Autodesk Inventor part; units mm, degrees
ref_plane "YZ Plane" through (0, 0, 0) normal (1, 0, 0) x (0, 1, 0)
ref_plane "XZ Plane" through (0, 0, 0) normal (0, 1, 0) x (-1, 0, 0)
ref_plane "XY Plane" through (0, 0, 0) normal (0, 0, 1) x (1, 0, 0)
sketch "Sketch4" plane through (0, 0, 0) normal (0, 1, 0) x (-1, 0, 0)
  line L0 (-127, 215.9) -> (127, 215.9)
  line L1 (127, 215.9) -> (127, -215.9)
  line L2 (127, -215.9) -> (-127, -215.9)
  line L3 (-127, -215.9) -> (-127, 215.9)
  line L4 (-127, 215.9) -> (127, -215.9) construction
  line L5 (127, 215.9) -> (-127, -215.9) construction
  point P0 (0, 0)
  dimension "d6" = 431.8
  dimension "d7" = 254
extrude "Plate1" add sketch "Sketch4" against normal blind 6.35
sketch "Sketch5" plane through (120.65, 0, -215.9) normal (1, 0, 0) x (0, -1, 0)
  line L0 (0, 431.8) -> (0, 0)
  line L1 (0, 0) -> (76.2, 0)
  line L2 (76.2, 0) -> (76.2, 431.8)
  line L3 (76.2, 431.8) -> (0, 431.8)
edge flange "Flange1" height 76.2 angle 90 thickness 6.35 bend radius 7.9502 thickness toward (1, 0, 0) relief tear relief width 6.35 relief depth 3.175 corner gap 6.35 corner form 0 edges at (127, 0, 0) (-127, 0, 0) wall of the first edge with corners at (120.65, 0, 215.9) (120.65, 0, -215.9) (120.65, -76.2, -215.9) (120.65, -76.2, 215.9)
bend "Bend1"
corner "Corner1"
sketch "Sketch6" plane through (0, 0, 0) normal (0, 1, 0) x (1, 0, 0)
  circle A0 centre (0, 0) radius 29.083
  dimension "d19" = 58.166
extrude "Cut1" cut sketch "Sketch6" against normal blind 6.35
sketch "Sketch7" plane through (0, 0, 0) normal (0, 1, 0) x (1, 0, 0)
  line L0 (-41.275, -165.1) -> (41.275, -165.1)
  line L1 (41.275, -165.1) -> (41.275, 165.1)
  line L2 (41.275, 165.1) -> (-41.275, 165.1)
  line L3 (-41.275, 165.1) -> (-41.275, -165.1)
  line L4 (-41.275, -165.1) -> (41.275, 165.1) construction
  line L5 (41.275, -165.1) -> (-41.275, 165.1) construction
  line L6 (112.6998, 215.9) -> (-112.6998, 215.9)
  point P0 (0, 0)
  dimension "d22" = 82.55
  dimension "d23" = 50.8
hole "Hole1" at (-41.275, 0, 165.1) at (41.275, 0, 165.1) at (-41.275, 0, -165.1) at (41.275, 0, -165.1) direction (0, -1, 0) diameter 12.7 depth 6.35
fillet "Corner Round1" radius 25.4 4 edges at (-123.825, -76.2, 215.9) (123.825, -76.2, 215.9) (123.825, -76.2, -215.9) (-123.825, -76.2, -215.9)
equation "\"d20\" = Thickness"
equation "\"d29\" = Thickness"
equation "\"d8\" = Thickness"
equation "\"d9\" = BendReliefWidth"
equation "\"d10\" = BendReliefDepth"
equation "\"d11\" = MinimumRemnant"
equation "\"d12\" = TransitionRadius"
equation "\"d15\" = BendRadius"
equation "\"d16\" = CornerReliefSize"
equation "\"d17\" = GapSize"
equation "\"d18\" = JacobiRadiusSize"
equation "\"BendReliefWidth\" = Thickness"
equation "\"BendReliefDepth\" = 0.5 * Thickness"
equation "\"CornerReliefSize\" = 4 * Thickness"
equation "\"MinimumRemnant\" = 2 * Thickness"
equation "\"TransitionRadius\" = BendRadius"
equation "\"JacobiRadiusSize\" = Thickness"
equation "\"GapSize\" = Thickness"
properties part number "Gooseneck Model-1 Sheet-1" material "SS304"
Work out the finished part from the listing and answer in its coordinate system (mm). A direction names the side the tool comes from. Coordinates: 2 decimals unless noted, no trailing zeros. Loops run counter-clockwise (first coordinate to the right, second up) from the corner with the lowest first, then second, coordinate; pieces in that order, holes last. Notation, with made-up numbers: (39.5, 72.5) -> (64.5, 72.5) arc R5 ccw to (64.5, 77.5) -> close; hole circle Ø9 at (83.25, 79). An arc over 180 degrees is marked (long way). Write each question's results on one line, items separated by ' | '. Start each with the question number.
1) A flat-ended cylindrical pin translates along its axis: P1, Ø12, axis at x = 77, z = 42, coming from the -Y side. Find the tip coordinate at first contact, or state that the pin passes through.
2) For faces 5 (the cylindrical face through (47.474, -3.219, -166.477)), 6 (the flat face through (120.65, -45, 3)), determine the directions among +Z, -Z, +X, -X, +Y, -Y from which every point of the face is accessible in a straight line to the end or side of a thin tool.
3) Find section B-B on z = 0. Determine the outline of the cut face in (x, y).
4) Find section A-A on z = -165.1. Determine the outline of the cut face in (x, y) (3 decimals), then the cut area to 3 significant figures.
5) Find section C-C on y = -25.5. Determine the outline of the cut face in (x, z), then the cut area to 3 significant figures.
6) Find section D-D on x = 0. Determine the outline of the cut face in (y, z), then the cut area to 3 significant figures.
7) The mould has two halves that part along X. Classify faces 1 (the cylindrical face through (-43.182, -3.219, 171.157)), 2 (the cylindrical face through (-123.87, -68.56, -208.66)), 3 (the flat face through (-120.65, -45, -3)), 4 (the flat face through (-127, -46, -3)): pulls with the +X half, pulls with the -X half, needs draft (parallel to the pull), parting line crosses it, or undercut.
8) Consider line 1 along X through (y, z) = (-25.5, 5); line 2 along X through (y, z) = (-2, -165.1) (3 decimals); line 3 along Z through (x, y) = (0, -2.25). Determine where each line is inside the solid, lowest interval first.
Response values:
1) P1: stops at y = -6.35
2) face 5: +Y, -Y | face 6: +Z, -Z, -Y
3) outline: (-127, -76.2) -> (-120.65, -76.2) -> (-120.65, -14.3) arc R7.95 cw to (-112.7, -6.35) -> (-29.08, -6.35) -> (-29.08, 0) -> (-112.7, 0) arc R14.3 ccw to (-127, -14.3) -> close; (29.08, -6.35) -> (112.7, -6.35) arc R7.95 cw to (120.65, -14.3) -> (120.65, -76.2) -> (127, -76.2) -> (127, -14.3) arc R14.3 ccw to (112.7, 0) -> (29.08, 0) -> close
4) outline: (-127, -76.2) -> (-120.65, -76.2) -> (-120.65, -14.3) arc R7.95 cw to (-112.7, -6.35) -> (-47.625, -6.35) -> (-47.625, 0) -> (-112.7, 0) arc R14.3 ccw to (-127, -14.3) -> close; (-34.925, -6.35) -> (34.925, -6.35) -> (34.925, 0) -> (-34.925, 0) -> close; (47.625, -6.35) -> (112.7, -6.35) arc R7.95 cw to (120.65, -14.3) -> (120.65, -76.2) -> (127, -76.2) -> (127, -14.3) arc R14.3 ccw to (112.7, 0) -> (47.625, 0) -> close | area: 2,280 mm^2
5) outline: (-127, -215.9) -> (-120.65, -215.9) -> (-120.65, 215.9) -> (-127, 215.9) -> close; (120.65, -215.9) -> (127, -215.9) -> (127, 215.9) -> (120.65, 215.9) -> close | area: 5,480 mm^2
6) outline: (-6.35, -215.9) -> (0, -215.9) -> (0, -29.08) -> (-6.35, -29.08) -> close; (-6.35, 29.08) -> (0, 29.08) -> (0, 215.9) -> (-6.35, 215.9) -> close | area: 2,370 mm^2
7) face 1: undercut | face 2: needs draft | face 3: undercut | face 4: pulls with the -X half
8) line 1: x = -127 to -120.65, 120.65 to 127 | line 2: x = -119.994 to -47.625, -34.925 to 34.925, 47.625 to 119.994 | line 3: z = -215.9 to -29.08, 29.08 to 215.9
